```python
from build123d import *

# Parameters (mm, degrees)
SKETCH2_R           = 2.7813
BOSS_EXTRUDE1_DEPTH = 3.175
SKETCH3_W           = 177.8
SKETCH3_H           = 53.34
CUT_EXTRUDE1_DEPTH  = 3.175
SKETCH4_R           = 2.7813
CUT_EXTRUDE2_DEPTH  = 3.175


with BuildPart() as part:
    # Sketch2 → Boss-Extrude1 (new body)
    with BuildSketch(Plane(origin=(0, 0, 0), x_dir=(1, 0, 0), z_dir=(0, 1, 0))):
        with BuildLine():
            Line((-106.7689, -102.8065), (106.7689, -102.8065))
            ThreePointArc((106.7689, -102.8065), (121.927572332, -96.527572332), (128.2065, -81.3689))
            Line((128.2065, -81.3689), (128.2065, 81.3689))
            ThreePointArc((128.2065, 81.3689), (121.927572332, 96.527572332), (106.7689, 102.8065))
            Line((106.7689, 102.8065), (-106.7689, 102.8065))
            ThreePointArc((-106.7689, 102.8065), (-121.927572332, 96.527572332), (-128.2065, 81.3689))
            Line((-128.2065, 81.3689), (-128.2065, -81.3689))
            ThreePointArc((-128.2065, -81.3689), (-121.927572332, -96.527572332), (-106.7689, -102.8065))
        make_face()
        with Locations((42.1132, 95.7453)):
            Circle(SKETCH2_R, mode=Mode.SUBTRACT)
        with Locations((117.221, 92.2909)):
            Circle(SKETCH2_R, mode=Mode.SUBTRACT)
        with Locations((120.4468, -3.3147)):
            Circle(SKETCH2_R, mode=Mode.SUBTRACT)
        with Locations((117.6274, -92.5195)):
            Circle(SKETCH2_R, mode=Mode.SUBTRACT)
        with Locations((49.403, -95.3643)):
            Circle(SKETCH2_R, mode=Mode.SUBTRACT)
        with Locations((-49.403, -95.3643)):
            Circle(SKETCH2_R, mode=Mode.SUBTRACT)
        with Locations((-117.6274, -92.5195)):
            Circle(SKETCH2_R, mode=Mode.SUBTRACT)
        with Locations((-120.4468, -3.3147)):
            Circle(SKETCH2_R, mode=Mode.SUBTRACT)
        with Locations((-117.221, 92.2909)):
            Circle(SKETCH2_R, mode=Mode.SUBTRACT)
        with Locations((-42.1132, 95.7453)):
            Circle(SKETCH2_R, mode=Mode.SUBTRACT)
    extrude(amount=BOSS_EXTRUDE1_DEPTH)

    # Sketch3 → Cut-Extrude1 (cut)
    with BuildSketch(Plane(origin=(0, 0, 0), x_dir=(1, 0, 0), z_dir=(0, 1, 0))):
        with Locations((0, -50.8)):
            Rectangle(SKETCH3_W, SKETCH3_H)
    extrude(amount=CUT_EXTRUDE1_DEPTH, mode=Mode.SUBTRACT)

    # Sketch4 → Cut-Extrude2 (cut)
    with BuildSketch(Plane(origin=(0, 0, 0), x_dir=(1, 0, 0), z_dir=(0, 1, 0))):
        with Locations((-95.25, -17.78)):
            Circle(SKETCH4_R)
        with Locations((0, -17.78)):
            Circle(SKETCH4_R)
        with Locations((95.25, -17.78)):
            Circle(SKETCH4_R)
        with Locations((95.25, -83.82)):
            Circle(SKETCH4_R)
        with Locations((0, -83.82)):
            Circle(SKETCH4_R)
        with Locations((-95.25, -83.82)):
            Circle(SKETCH4_R)
    extrude(amount=CUT_EXTRUDE2_DEPTH, mode=Mode.SUBTRACT)


solid = part.part
```
Geometry: final body of the model. Coordinates: model frame, mm. Round coordinates to 2 decimals unless told otherwise and drop trailing zeros. Write each loop counter-clockwise with the first axis right and the second up, starting at its lowest first coordinate (ties: lowest second). Pieces come first, ordered by that corner, then holes. Notation, with made-up numbers: (81.25, 19) -> (124.25, 19) arc R20 ccw to (124.25, 57) -> close; hole circle Ø7 at (81, 9.5). An arc over 180 degrees is marked (long way). Use CSV: the item, a comma, the result in double quotes. Start each with the question number.
Q1. Line query: L1, parallel to Z at x = -58.5, y = 0.65; L2, parallel to Z at x = -43.5, y = 0.65; L3, parallel to Z at x = -2, y = 1.35. Output: solid intervals per line, ascending.
Q2. Section C-C (x = 95.25). Return loops of the section in (y, z) (1 decimal).
Q3. Section A-A (x = 9). Return loops of the section in (y, z) (1 decimal).
Q4. Pull-direction query (X, two-part tool) for faces 1 (the face through (-122.093, 1.565, 96.36)), 2 (the face through (-2, 0, -1)), 3 (the face through (-0.362, 1.565, 81.062)); classes: pulls with the +X half, pulls with the -X half, needs draft (parallel to the pull), parting line crosses it, or undercut.
Q5. Section D-D (z = 64.5). Return loops of the section in (x, y) (1 decimal).
Q6. Section B-B (z = 17.78). Return loops of the section in (x, y) (1 decimal).
Result sheet:
1,L1,"-102.81 to 24.13, 77.47 to 102.81"
1,L2,"-102.81 to -98.16, -93.33 to 24.13, 77.47 to 102.81"
1,L3,"-102.81 to 15.85, 19.71 to 24.13, 77.47 to 81.89, 85.75 to 102.81"
2,outline,"(0, -102.8) -> (3.2, -102.8) -> (3.2, 15) -> (0, 15) -> close; (0, 20.6) -> (3.2, 20.6) -> (3.2, 81) -> (0, 81) -> close; (0, 86.6) -> (3.2, 86.6) -> (3.2, 102.8) -> (0, 102.8) -> close"
3,outline,"(0, -102.8) -> (3.2, -102.8) -> (3.2, 24.1) -> (0, 24.1) -> close; (0, 77.5) -> (3.2, 77.5) -> (3.2, 102.8) -> (0, 102.8) -> close"
4,face 1,"pulls with the -X half"
4,face 2,"needs draft"
4,face 3,"undercut"
5,outline,"(-128.2, 0) -> (-88.9, 0) -> (-88.9, 3.2) -> (-128.2, 3.2) -> close; (88.9, 0) -> (128.2, 0) -> (128.2, 3.2) -> (88.9, 3.2) -> close"
6,outline,"(-128.2, 0) -> (-98, 0) -> (-98, 3.2) -> (-128.2, 3.2) -> close; (-92.5, 0) -> (-2.8, 0) -> (-2.8, 3.2) -> (-92.5, 3.2) -> close; (2.8, 0) -> (92.5, 0) -> (92.5, 3.2) -> (2.8, 3.2) -> close; (98, 0) -> (128.2, 0) -> (128.2, 3.2) -> (98, 3.2) -> close"
